Here's how the part is built. I have some questions about the finished solid (model axes, mm). A direction names the side the tool comes from. Give positions to 0.01 mm unless a question says otherwise; leave off trailing zeros. Loops run counter-clockwise (first coordinate to the right, second up) from the corner with the lowest first, then second, coordinate; pieces in that order, holes last. Notation, with made-up numbers: (20, 37) - (76, 37) arc R20 ccw to (76, 53) - close; hole circle Ø1 at (49.5, 65.5). An arc over 180 degrees is marked (long way). Use one line per item in the form item = value.
from build123d import *

# Parameters (mm, degrees)
SKETCH1_W           = 30
SKETCH1_H           = 19.75
BOSS_EXTRUDE1_DEPTH = 4
SKETCH2_W           = 30
SKETCH2_H           = 5.9
BOSS_EXTRUDE2_DEPTH = 1.601
SKETCH3_W           = 10
SKETCH3_H           = 3
BOSS_EXTRUDE3_DEPTH = 18.7
SKETCH4_W           = 10
SKETCH4_H           = 3
BOSS_EXTRUDE4_DEPTH = 17.099
SKETCH5_W           = 10
SKETCH5_H           = 3
BOSS_EXTRUDE5_DEPTH = 1.601
FILLET1_R           = 2
CUT_EXTRUDE1_REACH  = 43.181
SKETCH6_R           = 1.4224
CUT_EXTRUDE2_REACH  = 43.181
SKETCH7_R           = 1.4224
SKETCH8_W           = 10
SKETCH8_H           = 3
SKETCH8_W_2         = 9.9
SKETCH8_H_2         = 2.9
CUT_EXTRUDE3_DEPTH  = 17.099


with BuildPart() as part:
    # Sketch1 → Boss-Extrude1 (new body)
    with BuildSketch(Plane(origin=(0, 0, 0), x_dir=(1, 0, 0), z_dir=(0, 1, 0))):
        with Locations((15, 9.875)):
            Rectangle(SKETCH1_W, SKETCH1_H)
    extrude(amount=BOSS_EXTRUDE1_DEPTH)

    # Sketch2 → Boss-Extrude2 (add)
    with BuildSketch(Plane(origin=(0, 4, 0), x_dir=(1, 0, 0), z_dir=(0, 1, 0))):
        with Locations((15, 16.8)):
            Rectangle(SKETCH2_W, SKETCH2_H)
    extrude(amount=BOSS_EXTRUDE2_DEPTH)

    # Sketch3 → Boss-Extrude3 (add)
    with BuildSketch(Plane(origin=(0, 4, 0), x_dir=(1, 0, 0), z_dir=(0, 1, 0))):
        with Locations((5, 1.5)):
            Rectangle(SKETCH3_W, SKETCH3_H)
        with Locations((25, 1.5)):
            Rectangle(SKETCH3_W, SKETCH3_H)
    extrude(amount=BOSS_EXTRUDE3_DEPTH)

    # Sketch4 → Boss-Extrude4 (add)
    with BuildSketch(Plane(origin=(0, 5.601, 0), x_dir=(1, 0, 0), z_dir=(0, 1, 0))):
        with Locations((5, 18.25)):
            Rectangle(SKETCH4_W, SKETCH4_H)
        with Locations((25, 18.25)):
            Rectangle(SKETCH4_W, SKETCH4_H)
    extrude(amount=BOSS_EXTRUDE4_DEPTH)

    # Sketch5 → Boss-Extrude5 (add)
    with BuildSketch(Plane(origin=(0, 4, 0), x_dir=(1, 0, 0), z_dir=(0, 1, 0))):
        with Locations((15, 1.5)):
            Rectangle(SKETCH5_W, SKETCH5_H)
    extrude(amount=BOSS_EXTRUDE5_DEPTH)

    # Fillet1
    fillet1_edges = [part.edges().sort_by_distance(p)[0] for p in [
        (15, 0, -19.75),
        (30, 0, -9.875),
        (15, 0, 0),
        (10, 14.1505, -19.75),
        (5, 22.7, -19.75),
        (0, 0, -9.875),
        (15, 5.601, -19.75),
        (20, 14.1505, -19.75),
        (25, 22.7, -19.75),
        (0, 11.35, -19.75),
        (30, 11.35, -19.75),
    ]]
    fillet(fillet1_edges, radius=FILLET1_R)

    # Sketch6 → Cut-Extrude1 (cut, up to next)
    with BuildSketch(Plane.XY.offset(-16.75), mode=Mode.PRIVATE) as cut_extrude1_sk1:
        with Locations((5, 19.2)):
            Circle(SKETCH6_R)
    cut_extrude1_tool1 = extrude(cut_extrude1_sk1.sketch, amount=-CUT_EXTRUDE1_REACH, mode=Mode.PRIVATE) & part.part
    # Sketch6 → Cut-Extrude1 (cut, up to next)
    with BuildSketch(Plane.XY.offset(-16.75), mode=Mode.PRIVATE) as cut_extrude1_sk2:
        with Locations((25, 19.2)):
            Circle(SKETCH6_R)
    cut_extrude1_tool2 = extrude(cut_extrude1_sk2.sketch, amount=-CUT_EXTRUDE1_REACH, mode=Mode.PRIVATE) & part.part
    # Sketch6 → Cut-Extrude1 (cut, up to next)
    with BuildSketch(Plane.XY.offset(-16.75), mode=Mode.PRIVATE) as cut_extrude1_sk3:
        with Locations((5, 14.2)):
            Circle(SKETCH6_R)
    cut_extrude1_tool3 = extrude(cut_extrude1_sk3.sketch, amount=-CUT_EXTRUDE1_REACH, mode=Mode.PRIVATE) & part.part
    # Sketch6 → Cut-Extrude1 (cut, up to next)
    with BuildSketch(Plane.XY.offset(-16.75), mode=Mode.PRIVATE) as cut_extrude1_sk4:
        with Locations((25, 14.2)):
            Circle(SKETCH6_R)
    cut_extrude1_tool4 = extrude(cut_extrude1_sk4.sketch, amount=-CUT_EXTRUDE1_REACH, mode=Mode.PRIVATE) & part.part
    add(cut_extrude1_tool1.solids().sort_by_distance((5, 19.2, -16.75))[0], mode=Mode.SUBTRACT)
    add(cut_extrude1_tool2.solids().sort_by_distance((25, 19.2, -16.75))[0], mode=Mode.SUBTRACT)
    add(cut_extrude1_tool3.solids().sort_by_distance((5, 14.2, -16.75))[0], mode=Mode.SUBTRACT)
    add(cut_extrude1_tool4.solids().sort_by_distance((25, 14.2, -16.75))[0], mode=Mode.SUBTRACT)

    # Sketch7 → Cut-Extrude2 (cut, up to next)
    with BuildSketch(Plane(origin=(0, 0, -3), x_dir=(-1, 0, 0), z_dir=(0, 0, -1)), mode=Mode.PRIVATE) as cut_extrude2_sk1:
        with Locations(Location((-25, 19.2, 0), (0, 0, 180))):
            Circle(SKETCH7_R)
    cut_extrude2_tool1 = extrude(cut_extrude2_sk1.sketch, amount=-CUT_EXTRUDE2_REACH, mode=Mode.PRIVATE) & part.part
    # Sketch7 → Cut-Extrude2 (cut, up to next)
    with BuildSketch(Plane(origin=(0, 0, -3), x_dir=(-1, 0, 0), z_dir=(0, 0, -1)), mode=Mode.PRIVATE) as cut_extrude2_sk2:
        with Locations(Location((-5, 19.2, 0), (0, 0, 180))):
            Circle(SKETCH7_R)
    cut_extrude2_tool2 = extrude(cut_extrude2_sk2.sketch, amount=-CUT_EXTRUDE2_REACH, mode=Mode.PRIVATE) & part.part
    # Sketch7 → Cut-Extrude2 (cut, up to next)
    with BuildSketch(Plane(origin=(0, 0, -3), x_dir=(-1, 0, 0), z_dir=(0, 0, -1)), mode=Mode.PRIVATE) as cut_extrude2_sk3:
        with Locations(Location((-5, 14.2, 0), (0, 0, 180))):
            Circle(SKETCH7_R)
    cut_extrude2_tool3 = extrude(cut_extrude2_sk3.sketch, amount=-CUT_EXTRUDE2_REACH, mode=Mode.PRIVATE) & part.part
    # Sketch7 → Cut-Extrude2 (cut, up to next)
    with BuildSketch(Plane(origin=(0, 0, -3), x_dir=(-1, 0, 0), z_dir=(0, 0, -1)), mode=Mode.PRIVATE) as cut_extrude2_sk4:
        with Locations(Location((-25, 14.2, 0), (0, 0, 180))):
            Circle(SKETCH7_R)
    cut_extrude2_tool4 = extrude(cut_extrude2_sk4.sketch, amount=-CUT_EXTRUDE2_REACH, mode=Mode.PRIVATE) & part.part
    add(cut_extrude2_tool1.solids().sort_by_distance((25, 19.2, -3))[0], mode=Mode.SUBTRACT)
    add(cut_extrude2_tool2.solids().sort_by_distance((5, 19.2, -3))[0], mode=Mode.SUBTRACT)
    add(cut_extrude2_tool3.solids().sort_by_distance((5, 14.2, -3))[0], mode=Mode.SUBTRACT)
    add(cut_extrude2_tool4.solids().sort_by_distance((25, 14.2, -3))[0], mode=Mode.SUBTRACT)

    # Sketch8 → Cut-Extrude3 (cut)
    # profile 1 of 2: a face of its own
    with BuildSketch(Plane(origin=(0, 22.7, 0), x_dir=(1, 0, 0), z_dir=(0, 1, 0))):
        with Locations((5, 1.5)):
            Rectangle(SKETCH8_W, SKETCH8_H)
        with Locations((5, 1.5)):
            Rectangle(SKETCH8_W_2, SKETCH8_H_2, mode=Mode.SUBTRACT)
    # profile 2 of 2: a face of its own
    with BuildSketch(Plane(origin=(0, 22.7, 0), x_dir=(1, 0, 0), z_dir=(0, 1, 0))):
        with Locations((25, 1.5)):
            Rectangle(SKETCH8_W, SKETCH8_H)
        with Locations((25, 1.5)):
            Rectangle(SKETCH8_W_2, SKETCH8_H_2, mode=Mode.SUBTRACT)
    extrude(amount=-CUT_EXTRUDE3_DEPTH, mode=Mode.SUBTRACT)


solid = part.part
(1) If we section it at C-C (x = 25): Give the number of separate pieces and of enclosed holes in the cut face, plus the area to 3 significant figures.
Geometry says:
separate_pieces = 5
enclosed_holes = 0
area = 158 mm²
(2) If I drill on probe 1 along Y at (x, z) = (25, -1.95); probe 2 along X at (y, z) = (14.2, -0.65); probe 3 along Y at (x, z) = (25, -1.55), over which ranges is the centre line in solid material (lowest first)?
Geometry says:
probe_1 = 0 to 12.78, 15.62 to 17.78, 20.62 to 22.7
probe_2 = 0.05 to 3.58, 6.42 to 9.95, 20.05 to 23.58, 26.42 to 29.95
probe_3 = 0.05 to 12.78, 15.62 to 17.78, 20.62 to 22.7
(3) If we section it at B-B (z = -17.25): List the corners of the cut face in (x, y) for me.
Geometry says:
outline = (0, 2) arc R2 ccw to (2, 0) - (28, 0) arc R2 ccw to (30, 2) - (30, 22.7) - (20, 22.7) - (20, 5.6) - (10, 5.6) - (10, 22.7) - (0, 22.7) - close; hole circle Ø2.84 at (5, 14.2); hole circle Ø2.84 at (5, 19.2); hole circle Ø2.84 at (25, 14.2); hole circle Ø2.84 at (25, 19.2)
(4) Thinking about a two-plate mould opening in X: for faces 1 (the flat face through (20.05, 14, -1)), 2 (the cylindrical face through (0.6, 12.21, -19.18)), 3 (the cylindrical face through (25.07, 22.13, -19.15)), which applies, pulls with the +X half, pulls with the -X half, needs draft (parallel to the pull), parting line crosses it, or undercut?
Geometry says:
face_1 = undercut
face_2 = pulls with the -X half
face_3 = needs draft
(5) For faces 4 (the flat face through (15, 5, -3)), 5 (the cylindrical face through (9.4, 13.28, -19.18)), 6 (the flat face through (0.05, 14, -1)), which set-ups out of +Z, -Z, +X, -X, +Y, -Y let a thin tool reach every point of the face, with its end or its side?
Geometry says:
face_4 = +X, -X, +Y
face_5 = -Z, +Y
face_6 = +Z, -X, +Y
(6) For P1, Ø1, axis at x = 6.5, z = -14.5, coming from the +Y side; P2, Ø2.5, axis at x = 5, y = 14.2, coming from the +Z side; P3, Ø0.8, axis at x = 19, y = 5, coming from the -Z side; P4, Ø2.5, axis at y = 13.5, z = -1.5, coming from the -X side, each with a flat end and sliding along its axis, tell me the tip position at first contact or that it passes through.
Geometry says:
P1 = 5.6
P2 = through
P3 = -19.48
P4 = 0.05
(7) If we section it at A-A (y = 12.25): List the corners of the cut face in (x, z) for me, plus the area to 3 significant figures.
Geometry says:
outline = (0, -17.75) arc R2 ccw to (2, -19.75) - (8, -19.75) arc R2 ccw to (10, -17.75) - (10, -16.75) - (0, -16.75) - close; (0.05, -2.95) - (9.95, -2.95) - (9.95, -0.05) - (0.05, -0.05) - close; (20, -17.75) arc R2 ccw to (22, -19.75) - (28, -19.75) arc R2 ccw to (30, -17.75) - (30, -16.75) - (20, -16.75) - close; (20.05, -2.95) - (29.95, -2.95) - (29.95, -0.05) - (20.05, -0.05) - close
area = 114 mm²
(8) If we section it at D-D (z = -14.5): List the corners of the cut face in (x, y) for me, plus the area to 3 significant figures.
Geometry says:
outline = (0, 2) arc R2 ccw to (2, 0) - (28, 0) arc R2 ccw to (30, 2) - (30, 5.6) - (0, 5.6) - close
area = 166 mm²
